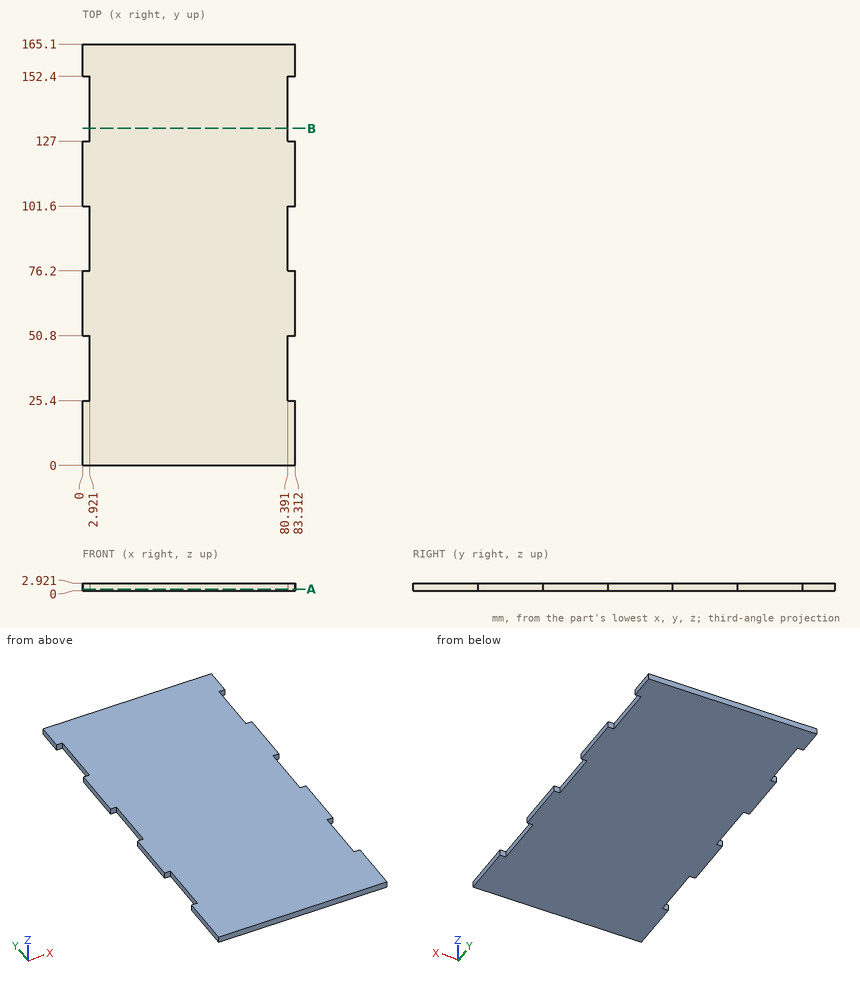
Design review of the part shown in the three views and the two pictorial views. Dimensions are in mm from the part's minimum x, y and z. Give positions to 0.01 mm unless a question says otherwise; leave off trailing zeros. Loops run counter-clockwise (first coordinate to the right, second up) from the corner with the lowest first, then second, coordinate; pieces in that order, holes last. Notation, with made-up numbers: M 33,54 L 65,54 A29 cw 65,88 Z; hole C 54.25,63 d2. An arc over 180 degrees is marked long. Put each result on its own line as item: value. Start each with the question number.
(1) For pin 1 (1.5 mm diameter, centred on y = 142.5, z = 1, fed in from -X); pin 2 (0.9 mm diameter, centred on y = 33.5, z = 1, fed in from +X), all flat-tipped, find the tip position at first contact; note any pin that passes through.
(2) Wall thickness on L1, parallel to X at y = 30.5, z = 0.7: over which ranges is the line inside the solid? List them lowest first.
(3) Add section A-A, the plane z = 0.65. Write out the cut boundary in (x, y), then the cut area to 3 significant figures.
(4) Add section B-B, the plane y = 132. Write out the cut boundary in (x, z).
Result:
1. pin 1: stops at x = 2.92
1. pin 2: stops at x = 80.39
2. L1: x = 2.92 to 80.39
3. outline: M 0,0 L 83.31,0 L 83.31,25.4 L 80.39,25.4 L 80.39,50.8 L 83.31,50.8 L 83.31,76.2 L 80.39,76.2 L 80.39,101.6 L 83.31,101.6 L 83.31,127 L 80.39,127 L 80.39,152.4 L 83.31,152.4 L 83.31,165.1 L 0,165.1 L 0,152.4 L 2.92,152.4 L 2.92,127 L 0,127 L 0,101.6 L 2.92,101.6 L 2.92,76.2 L 0,76.2 L 0,50.8 L 2.92,50.8 L 2.92,25.4 L 0,25.4 Z
3. area: 13,300 mm^2
4. outline: M 2.92,0 L 80.39,0 L 80.39,2.92 L 2.92,2.92 Z
